Read the model definition and answer for the solid it produces. Units are mm, in the model's axes. A direction names the side the tool comes from. Round coordinates to 2 decimals unless told otherwise and drop trailing zeros. Loops run counter-clockwise (first coordinate to the right, second up) from the corner with the lowest first, then second, coordinate; pieces in that order, holes last. Notation, with made-up numbers: M 59.25,66 L 87.25,66 A22 ccw 87.25,98 Z; hole C 39.25,-29.75 d6. An arc over 180 degrees is marked long. Write each question's results on one line, items separated by ' | '.
```python
from build123d import *

# Parameters (mm, degrees)
BOSS_EXTRU_1_DEPTH      = 25
ESQUISSE2_R             = 1.55
ENL_V_MAT_EXTRU_1_DEPTH = 28.477263328
ENL_V_START             = -3
ESQUISSE3_R             = 1.9
ENL_V_MAT_EXTRU_2_DEPTH = 25.477263328
ESQUISSE4_R             = 3.5
ESQUISSE4_R_2           = 1.9
BOSS_EXTRU_2_DEPTH      = 8
ENL_V_MAT_EXTRU_3_DEPTH = 15
ESQUISSE7_R             = 1.55
ENL_V_MAT_EXTRU_4_DEPTH = 28.748873851
ENL_V_START_2           = -2
ESQUISSE8_R             = 1.9
ENL_V_MAT_EXTRU_5_DEPTH = 26.748873851
CONG_1_R                = 1
CONG_2_START            = -26
CONG_2_DEPTH            = 52


with BuildPart() as part:
    # Esquisse1 → Boss.-Extru.1 (new, symmetric)
    with BuildSketch(Plane(origin=(0, 0, 0), x_dir=(0, 0, -1), z_dir=(1, 0, 0))):
        Polygon((0, 0), (9, 0), (9, 7), (-1.875644347, 7), align=None)
    extrude(amount=BOSS_EXTRU_1_DEPTH, both=True)

    # Esquisse2 → Enlèv. mat.-Extru.1 (cut, through all)
    with BuildSketch(Plane.XZ):
        with Locations(Location((-21, -4.4, 0), (0, 0, 270))):
            Circle(ESQUISSE2_R)
        with Locations(Location((21, -4.4, 0), (0, 0, 90))):
            Circle(ESQUISSE2_R)
    extrude(amount=-ENL_V_MAT_EXTRU_1_DEPTH, mode=Mode.SUBTRACT)

    # Esquisse3 → Enlèv. mat.-Extru.2 (cut, through all)
    with BuildSketch(Plane.XZ.offset(ENL_V_START)):
        with Locations(Location((-21, -4.4, 0), (0, 0, 270))):
            Circle(ESQUISSE3_R)
        with Locations(Location((21, -4.4, 0), (0, 0, 270))):
            Circle(ESQUISSE3_R)
    extrude(amount=-ENL_V_MAT_EXTRU_2_DEPTH, mode=Mode.SUBTRACT)

    # Esquisse4 → Boss.-Extru.2 (add)
    # profile 1 of 2: a face of its own
    with BuildSketch(Plane(origin=(0, 0, 0), x_dir=(1, 0, 0), z_dir=(0, 1, 0))):
        with Locations(Location((-21, 4.4, 0), (0, 0, 90))):
            Circle(ESQUISSE4_R)
        with Locations(Location((-21, 4.4, 0), (0, 0, 90))):
            Circle(ESQUISSE4_R_2, mode=Mode.SUBTRACT)
    # profile 2 of 2: a face of its own
    with BuildSketch(Plane(origin=(0, 0, 0), x_dir=(1, 0, 0), z_dir=(0, 1, 0))):
        with Locations(Location((21, 4.4, 0), (0, 0, 90))):
            Circle(ESQUISSE4_R)
        with Locations(Location((21, 4.4, 0), (0, 0, 90))):
            Circle(ESQUISSE4_R_2, mode=Mode.SUBTRACT)
    extrude(amount=BOSS_EXTRU_2_DEPTH)

    # Esquisse6 → Enlèv. mat.-Extru.3 (cut, symmetric)
    with BuildSketch(Plane(origin=(0, 0, 0), x_dir=(0, 0, -1), z_dir=(1, 0, 0))):
        Polygon((3.300736555, 7), (4.747662194, 1.6), (9, 1.6), (9, 7), align=None)
    extrude(amount=ENL_V_MAT_EXTRU_3_DEPTH, both=True, mode=Mode.SUBTRACT)

    # Esquisse7 → Enlèv. mat.-Extru.4 (cut, through all)
    with BuildSketch(Plane(origin=(0, 0, 0), x_dir=(1, 0, 0), z_dir=(0, -0.25881904510252496, 0.9659258262890672))):
        with Locations(Location((0, 2.5, 0), (0, 0, 270))):
            Circle(ESQUISSE7_R)
    extrude(amount=-ENL_V_MAT_EXTRU_4_DEPTH, mode=Mode.SUBTRACT)

    # Esquisse8 → Enlèv. mat.-Extru.5 (cut, through all)
    with BuildSketch(Plane(origin=(0, 0, 0), x_dir=(1, 0, 0), z_dir=(0, -0.25881904510252496, 0.9659258262890672)).offset(ENL_V_START_2)):
        with Locations(Location((0, 2.5, 0), (0, 0, 270))):
            Circle(ESQUISSE8_R)
    extrude(amount=-ENL_V_MAT_EXTRU_5_DEPTH, mode=Mode.SUBTRACT)

    # Congé1
    cong_1_edges = [part.edges().sort_by_distance(p)[0] for p in [
        (25, 3.5, -9),
        (-21, 7, -0.9),
        (25, 3.5, 0.937822174),
        (21, 7, -0.9),
        (-25, 3.5, -9),
        (-25, 3.5, 0.937822174),
        (-15, 4.3, -9),
        (-15, 4.3, -4.024199375),
        (15, 4.3, -9),
        (15, 4.3, -4.024199375),
    ]]
    fillet(cong_1_edges, radius=CONG_1_R - 0.0001)  # a hair under: the kernel refuses the full size

    # Congé2: read off the stored shape, not the designer's step
    # Congé2 outline → Congé2 (cut)
    with BuildSketch(Plane.YZ.offset(CONG_2_START)):
        with BuildLine():
            Line((7, 1.875644347), (5.741180955, 1.5383448))
            ThreePointArc((5.741180955, 1.5383448), (6.608761429, 1.365772314), (7, 0.572418974))
            Line((7, 0.572418974), (7, 1.875644347))
        make_face()
    extrude(amount=CONG_2_DEPTH, mode=Mode.SUBTRACT)


solid = part.part
```
1. Determine the mould class of faces 1 (the face through (24.699, 3.249, 0.575)), 2 (the face through (19.116, 5.465, -4.153)), 3 (the face through (23, 8, -6)) for opening direction Z: released by +Z, released by -Z, zero draft, split by the parting line, or undercut.
Completed:
face 1: released by +Z | face 2: undercut | face 3: zero draft
2. Given P1, Ø1, axis at x = -8.5, z = -3, coming from the +Y side; P2, Ø3, axis at x = -12.5, z = -7, coming from the +Y side; P3, Ø1.5, axis at x = 14, y = 2, coming from the +Z side, each flat-ended and moving along its own axis, determine where each tip first touches the part or whether it passes through.
Completed:
P1: stops at y = 7 | P2: stops at y = 1.6 | P3: stops at z = 0.74
3. Find the intervals of material crossed by L1, parallel to X at y = 1.5, z = -4.4; L2, parallel to X at y = 6.2, z = -4.4; L3, parallel to X at y = 5.1, z = -4.4, in increasing order.
Completed:
L1: x = -25 to -22.55, -19.45 to 19.45, 22.55 to 25 | L2: x = -25 to -22.9, -19.1 to -14.99, 14.99 to 19.1, 22.9 to 25 | L3: x = -25 to -22.9, -19.1 to -14.9, 14.9 to 19.1, 22.9 to 25
4. Find section B-B, the plane x = 10.5. Give the vertices of the cut face in (y, z), then the cut area to 3 significant figures.
Completed:
outline: M 0,-9 L 1.6,-9 L 1.6,-4.75 L 7,-3.3 L 7,0.57 A1 ccw 5.74,1.54 L 0,0 Z | area: 42.3 mm2
5. Which of the six approach directions +Z, -Z, +X, -X, +Y, -Y give full straight-line access (tool end or side, diameter ignored) to faces 4 (the face through (0.336, 4.187, 1.122)), 5 (the face through (-15, 4, -7))?
Completed:
face 4: +Z, +X, -X, -Y | face 5: -Z, +Y
6. Find section C-C, the plane y = 3.5. Count the separate pieces of the cut face and the enclosed holes in it, then the cut area to 3 significant figures.
Completed:
separate pieces: 2 | enclosed holes: 2 | area: 314 mm2
